Answer from the drawing. Dimensions are ordinates in mm from the lowest x, y and z of the part. Round coordinates to 2 decimals unless told otherwise and drop trailing zeros. Write each loop counter-clockwise with the first axis right and the second up, starting at its lowest first coordinate (ties: lowest second). Pieces come first, ordered by that corner, then holes. Notation, with made-up numbers: (49.25, -16.5) -> (55.25, -16.5) arc R19 cw to (55.25, 15.5) -> close; hole circle Ø4 at (7.5, 86). An arc over 180 degrees is marked (long way). Return JSON: item names as keys, results as strings. Group by question number.
(1) A cutting plane is placed at C-C on y = 2. Give the vertices of the cut face in (x, z).
(2) Straight lines are drawn through the part: line 1 (Z direction, x = 44, y = 2); line 2 (X direction, y = 3.5, z = 7); line 3 (X direction, y = 7.25, z = 8.5). For each, find the intervals that lie inside material, in ascending order.
(3) A cutting plane is placed at A-A on z = 7.5. Give the vertices of the cut face in (x, y), then the cut area to 3 significant figures.
(4) A cutting plane is placed at B-B on x = 44. Give the vertices of the cut face in (y, z), then the cut area to 3 significant figures.
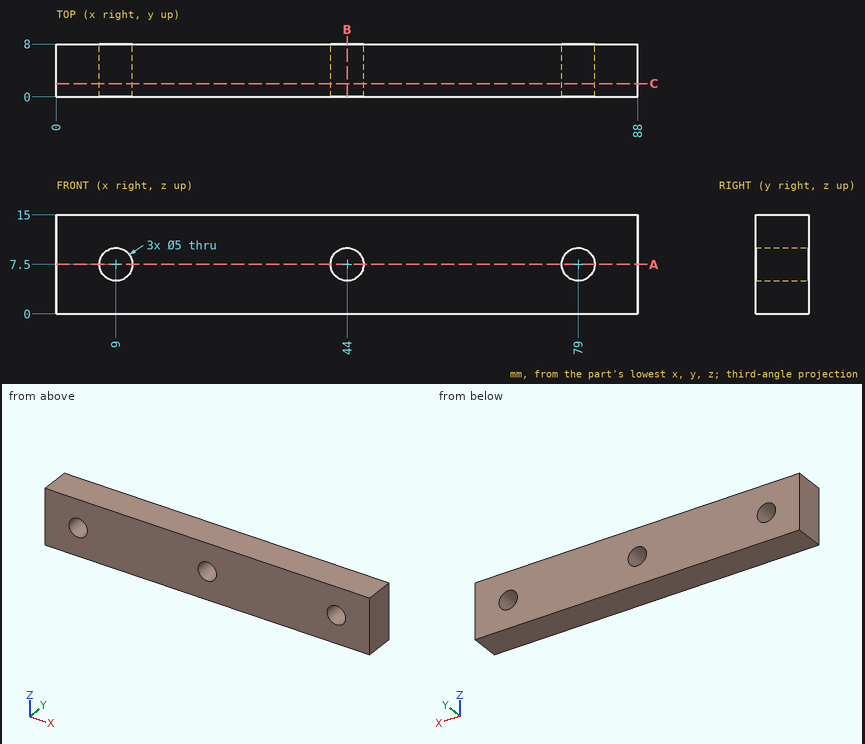
Checks:
{
 "1": {"outline": "(0, 0) -> (88, 0) -> (88, 15) -> (0, 15) -> close; hole circle Ø5 at (9, 7.5); hole circle Ø5 at (44, 7.5); hole circle Ø5 at (79, 7.5)"},
 "2": {"line 1": "z = 0 to 5, 10 to 15", "line 2": "x = 0 to 6.55, 11.45 to 41.55, 46.45 to 76.55, 81.45 to 88", "line 3": "x = 0 to 6.71, 11.29 to 41.71, 46.29 to 76.71, 81.29 to 88"},
 "3": {"outline": "(0, 0) -> (6.5, 0) -> (6.5, 8) -> (0, 8) -> close; (11.5, 0) -> (41.5, 0) -> (41.5, 8) -> (11.5, 8) -> close; (46.5, 0) -> (76.5, 0) -> (76.5, 8) -> (46.5, 8) -> close; (81.5, 0) -> (88, 0) -> (88, 8) -> (81.5, 8) -> close", "area": "584 mm^2"},
 "4": {"outline": "(0, 0) -> (8, 0) -> (8, 5) -> (0, 5) -> close; (0, 10) -> (8, 10) -> (8, 15) -> (0, 15) -> close", "area": "80.0 mm^2"}
}
